Could you check a few things on this drawing? It's one solid part, dimensions in mm from its lowest x, y, z. Round coordinates to 2 decimals unless told otherwise and drop trailing zeros. Order: outer loops, then holes, each group sorted by start corner. A loop starts at its lowest first (then second) coordinate and runs counter-clockwise, first axis right, second up.
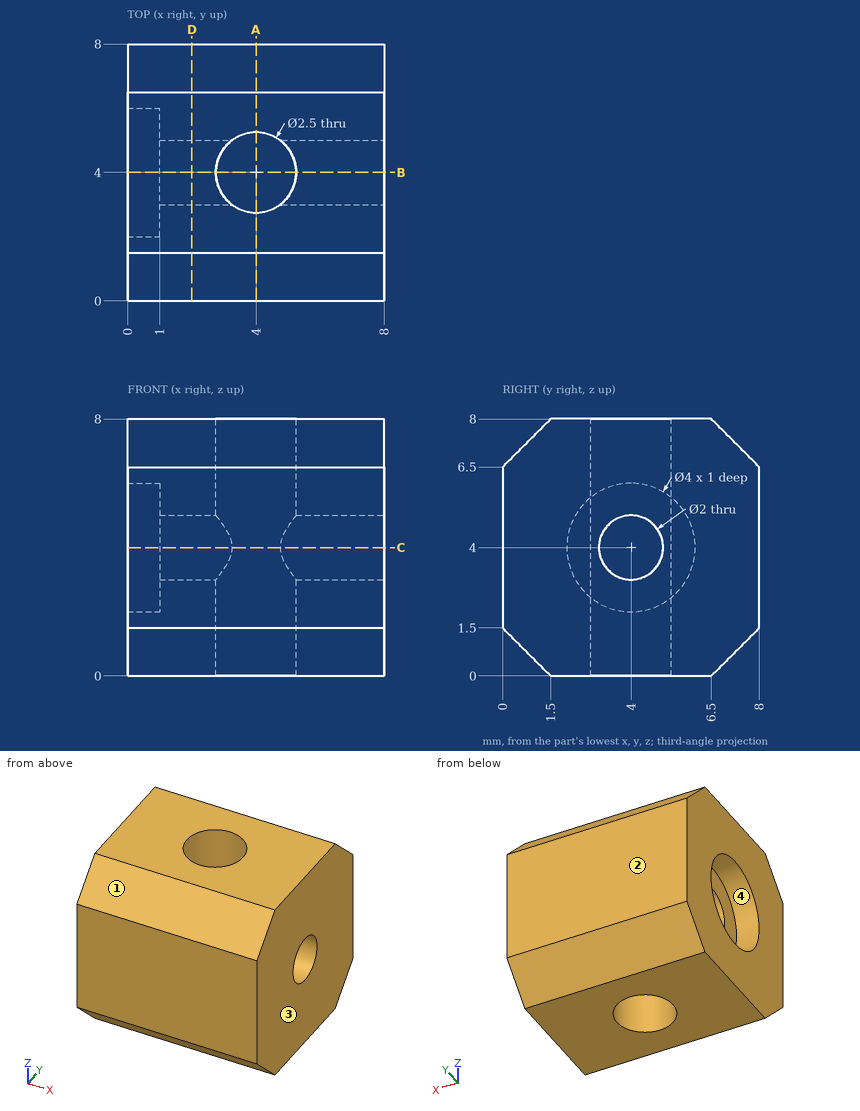
1) I'm going to push flat-ended pins straight in: pin 1 (3 mm diameter, centred on y = 6.5, z = 1, fed in from -X); pin 2 (2.5 mm diameter, centred on y = 4, z = 4, fed in from -X). Where does each tip first touch, or does it pass through?
2) If we section it at C-C (z = 4): Write out the boundary of the cut face in (x, y).
3) I need wall thicknesses on line 1 (Y direction, x = 7, z = 4); line 2 (X direction, y = 3, z = 3.25). Which ranges of each line are inside material? Lowest first, please.
4) If we section it at D-D (x = 2): Write out the boundary of the cut face in (y, z).
5) If we section it at A-A (x = 4): Write out the boundary of the cut face in (y, z), plus the area to 3 significant figures.
6) If we section it at B-B (y = 4): Write out the boundary of the cut face in (x, z), plus the area to 3 significant figures.
7) We'd pull the mould along Y, two halves only. Please class the marked faces 1, 2, 3 and 4: +Y half, -Y half, draft (parallel to the pull), parting line (faces both ways), or undercut.
Solutions:
1. pin 1: stops at x = 0
1. pin 2: stops at x = 1
2. outline: (0, 0) - (8, 0) - (8, 3) - (4.75, 3) arc R1.25 cw to (3.25, 3) - (1, 3) - (1, 2) - (0, 2) - close; (0, 6) - (1, 6) - (1, 5) - (3.25, 5) arc R1.25 cw to (4.75, 5) - (8, 5) - (8, 8) - (0, 8) - close
3. line 1: y = 0 to 3, 5 to 8
3. line 2: x = 1 to 3.25, 4.75 to 8
4. outline: (0, 1.5) - (1.5, 0) - (6.5, 0) - (8, 1.5) - (8, 6.5) - (6.5, 8) - (1.5, 8) - (0, 6.5) - close; hole circle Ø2 at (4, 4)
5. outline: (0, 1.5) - (1.5, 0) - (2.75, 0) - (2.75, 8) - (1.5, 8) - (0, 6.5) - close; (5.25, 0) - (6.5, 0) - (8, 1.5) - (8, 6.5) - (6.5, 8) - (5.25, 8) - close
5. area: 39.5 mm2
6. outline: (0, 0) - (2.75, 0) - (2.75, 3) - (1, 3) - (1, 2) - (0, 2) - close; (0, 6) - (1, 6) - (1, 5) - (2.75, 5) - (2.75, 8) - (0, 8) - close; (5.25, 0) - (8, 0) - (8, 3) - (5.25, 3) - close; (5.25, 5) - (8, 5) - (8, 8) - (5.25, 8) - close
6. area: 31.0 mm2
7. face 1: -Y half
7. face 2: +Y half
7. face 3: draft
7. face 4: undercut
